Verification items for the finished model (mm, model axes). Give positions to 0.01 mm unless a question says otherwise; leave off trailing zeros. Order: outer loops, then holes, each group sorted by start corner. A loop starts at its lowest first (then second) coordinate and runs counter-clockwise, first axis right, second up. Notation, with made-up numbers: (11, 54.5) -> (27, 54.5) arc R25 ccw to (27, 82.5) -> close; hole circle Ø5 at (57, -6.5). An arc over 180 degrees is marked (long way). One line per question, with ' | ' between items. Start each with the question number.
Q1. Go/stop test with flat-tipped pins: pin 1 (6 mm diameter, centred on y = 7, z = -3, fed in from -X); pin 2 (6 mm diameter, centred on x = -57, y = 10.5, fed in from +Z); pin 3 (3 mm diameter, centred on x = -18.5, z = 7.5, fed in from +Y). Record where each tip stops, or that it passes through.
Q2. Mould release check, pull along Y, two halves, no side actions. Record for faces 1 (the flat face through (-1, 1, -25.4)), 2 (the cylindrical face through (52.37, -0.04, 3.95)): released by +Y, released by -Y, zero draft, split by the parting line, or undercut.
Q3. Material ranges on probe 1 along X at (y, z) = (-65, 2.5); probe 2 along Z at (x, y) = (-18.5, -31); probe 3 along X at (y, z) = (40.5, -5), recorded low to high. Write a range as [from, to].
Q4. Section check B-B on z = -15. Record the cut outline in (x, y).
from build123d import *

# Parameters (mm, degrees)
F0_R          = 76.2
F1_DEPTH      = 25.4
F4_DEPTH      = 20.21225
F4_DEPTH_BACK = 6.35


with BuildPart() as f1:
    # F0 (on Top) → F1 (new body)
    with BuildSketch(Plane.XY):
        Circle(F0_R)
        with BuildLine():
            ThreePointArc((-15.062988, 32.279811), (-13.412606, 32.380894), (-12.174132, 33.476414))
            Line((-12.174132, 33.476414), (-2.210489, 51.080058))
            ThreePointArc((-2.210489, 51.080058), (0, 52.368924), (2.210489, 51.080058))
            Line((2.210489, 51.080058), (12.174132, 33.476414))
            ThreePointArc((12.174132, 33.476414), (13.412606, 32.380894), (15.062988, 32.279811))
            Line((15.062988, 32.279811), (34.556004, 37.682107))
            ThreePointArc((34.556004, 37.682107), (37.030421, 37.030421), (37.682107, 34.556004))
            Line((37.682107, 34.556004), (32.279811, 15.062988))
            ThreePointArc((32.279811, 15.062988), (32.380894, 13.412606), (33.476414, 12.174132))
            Line((33.476414, 12.174132), (51.080058, 2.210489))
            ThreePointArc((51.080058, 2.210489), (52.368924, 0), (51.080058, -2.210489))
            Line((51.080058, -2.210489), (33.476414, -12.174132))
            ThreePointArc((33.476414, -12.174132), (32.380894, -13.412606), (32.279811, -15.062988))
            Line((32.279811, -15.062988), (37.682107, -34.556004))
            ThreePointArc((37.682107, -34.556004), (37.030421, -37.030421), (34.556004, -37.682107))
            Line((34.556004, -37.682107), (15.062988, -32.279811))
            ThreePointArc((15.062988, -32.279811), (13.412606, -32.380894), (12.174132, -33.476414))
            Line((12.174132, -33.476414), (2.210489, -51.080058))
            ThreePointArc((2.210489, -51.080058), (0, -52.368924), (-2.210489, -51.080058))
            Line((-2.210489, -51.080058), (-12.174132, -33.476414))
            ThreePointArc((-12.174132, -33.476414), (-13.412606, -32.380894), (-15.062988, -32.279811))
            Line((-15.062988, -32.279811), (-34.556004, -37.682107))
            ThreePointArc((-34.556004, -37.682107), (-37.030421, -37.030421), (-37.682107, -34.556004))
            Line((-37.682107, -34.556004), (-32.279811, -15.062988))
            ThreePointArc((-32.279811, -15.062988), (-32.380894, -13.412606), (-33.476414, -12.174132))
            Line((-33.476414, -12.174132), (-51.080058, -2.210489))
            ThreePointArc((-51.080058, -2.210489), (-52.368924, 0), (-51.080058, 2.210489))
            Line((-51.080058, 2.210489), (-33.476414, 12.174132))
            ThreePointArc((-33.476414, 12.174132), (-32.380894, 13.412606), (-32.279811, 15.062988))
            Line((-32.279811, 15.062988), (-37.682107, 34.556004))
            ThreePointArc((-37.682107, 34.556004), (-37.030421, 37.030421), (-34.556004, 37.682107))
            Line((-34.556004, 37.682107), (-15.062988, 32.279811))
        make_face(mode=Mode.SUBTRACT)
        with BuildLine():
            Line((-2.210489, 51.080058), (-12.174132, 33.476414))
            ThreePointArc((-12.174132, 33.476414), (-13.412606, 32.380894), (-15.062988, 32.279811))
            Line((-15.062988, 32.279811), (-34.556004, 37.682107))
            ThreePointArc((-34.556004, 37.682107), (-37.030421, 37.030421), (-37.682107, 34.556004))
            Line((-37.682107, 34.556004), (-32.279811, 15.062988))
            ThreePointArc((-32.279811, 15.062988), (-32.380894, 13.412606), (-33.476414, 12.174132))
            Line((-33.476414, 12.174132), (-51.080058, 2.210489))
            ThreePointArc((-51.080058, 2.210489), (-52.368924, 0), (-51.080058, -2.210489))
            Line((-51.080058, -2.210489), (-33.476414, -12.174132))
            ThreePointArc((-33.476414, -12.174132), (-32.380894, -13.412606), (-32.279811, -15.062988))
            Line((-32.279811, -15.062988), (-37.682107, -34.556004))
            ThreePointArc((-37.682107, -34.556004), (-37.030421, -37.030421), (-34.556004, -37.682107))
            Line((-34.556004, -37.682107), (-15.062988, -32.279811))
            ThreePointArc((-15.062988, -32.279811), (-13.412606, -32.380894), (-12.174132, -33.476414))
            Line((-12.174132, -33.476414), (-2.210489, -51.080058))
            ThreePointArc((-2.210489, -51.080058), (0, -52.368924), (2.210489, -51.080058))
            Line((2.210489, -51.080058), (12.174132, -33.476414))
            ThreePointArc((12.174132, -33.476414), (13.412606, -32.380894), (15.062988, -32.279811))
            Line((15.062988, -32.279811), (34.556004, -37.682107))
            ThreePointArc((34.556004, -37.682107), (37.030421, -37.030421), (37.682107, -34.556004))
            Line((37.682107, -34.556004), (32.279811, -15.062988))
            ThreePointArc((32.279811, -15.062988), (32.380894, -13.412606), (33.476414, -12.174132))
            Line((33.476414, -12.174132), (51.080058, -2.210489))
            ThreePointArc((51.080058, -2.210489), (52.368924, 0), (51.080058, 2.210489))
            Line((51.080058, 2.210489), (33.476414, 12.174132))
            ThreePointArc((33.476414, 12.174132), (32.380894, 13.412606), (32.279811, 15.062988))
            Line((32.279811, 15.062988), (37.682107, 34.556004))
            ThreePointArc((37.682107, 34.556004), (37.030421, 37.030421), (34.556004, 37.682107))
            Line((34.556004, 37.682107), (15.062988, 32.279811))
            ThreePointArc((15.062988, 32.279811), (13.412606, 32.380894), (12.174132, 33.476414))
            Line((12.174132, 33.476414), (2.210489, 51.080058))
            ThreePointArc((2.210489, 51.080058), (0, 52.368924), (-2.210489, 51.080058))
        make_face()
    extrude(amount=-F1_DEPTH)

    # F2 (on Right) → F3 (revolve)
    with BuildSketch(Plane.YZ):
        with BuildLine():
            add(Edge.make_bspline(
                [(0, 20.21125), (-53.338584, 20.21125), (-76.2, 6.136773), (-76.2, 0)],
                knots=[0, 0, 0, 0, 78.834857, 78.834857, 78.834857, 78.834857], degree=3))
            Line((-76.2, 0), (0, 0))
            Line((0, 0), (0, 20.21125))
        make_face()
    revolve(axis=Axis((0, 0, 10.105625), (0, 0, -1)))

    # F0 (on Top) → F4 (cut, two sides)
    with BuildSketch(Plane.XY) as f4_sk:
        with BuildLine():
            Line((-2.210489, 51.080058), (-12.174132, 33.476414))
            ThreePointArc((-12.174132, 33.476414), (-13.412606, 32.380894), (-15.062988, 32.279811))
            Line((-15.062988, 32.279811), (-34.556004, 37.682107))
            ThreePointArc((-34.556004, 37.682107), (-37.030421, 37.030421), (-37.682107, 34.556004))
            Line((-37.682107, 34.556004), (-32.279811, 15.062988))
            ThreePointArc((-32.279811, 15.062988), (-32.380894, 13.412606), (-33.476414, 12.174132))
            Line((-33.476414, 12.174132), (-51.080058, 2.210489))
            ThreePointArc((-51.080058, 2.210489), (-52.368924, 0), (-51.080058, -2.210489))
            Line((-51.080058, -2.210489), (-33.476414, -12.174132))
            ThreePointArc((-33.476414, -12.174132), (-32.380894, -13.412606), (-32.279811, -15.062988))
            Line((-32.279811, -15.062988), (-37.682107, -34.556004))
            ThreePointArc((-37.682107, -34.556004), (-37.030421, -37.030421), (-34.556004, -37.682107))
            Line((-34.556004, -37.682107), (-15.062988, -32.279811))
            ThreePointArc((-15.062988, -32.279811), (-13.412606, -32.380894), (-12.174132, -33.476414))
            Line((-12.174132, -33.476414), (-2.210489, -51.080058))
            ThreePointArc((-2.210489, -51.080058), (0, -52.368924), (2.210489, -51.080058))
            Line((2.210489, -51.080058), (12.174132, -33.476414))
            ThreePointArc((12.174132, -33.476414), (13.412606, -32.380894), (15.062988, -32.279811))
            Line((15.062988, -32.279811), (34.556004, -37.682107))
            ThreePointArc((34.556004, -37.682107), (37.030421, -37.030421), (37.682107, -34.556004))
            Line((37.682107, -34.556004), (32.279811, -15.062988))
            ThreePointArc((32.279811, -15.062988), (32.380894, -13.412606), (33.476414, -12.174132))
            Line((33.476414, -12.174132), (51.080058, -2.210489))
            ThreePointArc((51.080058, -2.210489), (52.368924, 0), (51.080058, 2.210489))
            Line((51.080058, 2.210489), (33.476414, 12.174132))
            ThreePointArc((33.476414, 12.174132), (32.380894, 13.412606), (32.279811, 15.062988))
            Line((32.279811, 15.062988), (37.682107, 34.556004))
            ThreePointArc((37.682107, 34.556004), (37.030421, 37.030421), (34.556004, 37.682107))
            Line((34.556004, 37.682107), (15.062988, 32.279811))
            ThreePointArc((15.062988, 32.279811), (13.412606, 32.380894), (12.174132, 33.476414))
            Line((12.174132, 33.476414), (2.210489, 51.080058))
            ThreePointArc((2.210489, 51.080058), (0, 52.368924), (-2.210489, 51.080058))
        make_face()
    extrude(amount=F4_DEPTH, mode=Mode.SUBTRACT)
    extrude(f4_sk.sketch, amount=-F4_DEPTH_BACK, mode=Mode.SUBTRACT)


solid = f1.part
Filled in:
1) pin 1: x = -76.09 | pin 2: z = 13.43 | pin 3: y = 69.04
2) face 1: zero draft | face 2: undercut
3) probe 1: [-37.83, 37.83] | probe 2: [-25.4, -6.35] | probe 3: [-64.55, -8.2], [8.2, 64.55]
4) outline: circle Ø152.4 at (0, 0)
